```python
from build123d import *

# Parameters (mm, degrees)
F0_W     = 47.4027246237
F0_H     = 29.581496492
F1_DEPTH = 25
F3_D     = 5.5
F3_DEPTH = 12
F3_TIP   = 1.6523667023
F5_D     = 5.5
F5_DEPTH = 12
F5_TIP   = 1.6523667023


with BuildPart() as f1:
    # F0 (on Front) → F1 (new body)
    with BuildSketch(Plane.XZ):
        with Locations((23.7013623118, 14.790748246)):
            Rectangle(F0_W, F0_H)
    extrude(amount=F1_DEPTH)

    # F3
    with Locations(Plane.XY.offset(29.581496492)):
        with Locations((23.7013623118, -12.5)):
            Hole(F3_D / 2, depth=F3_DEPTH)
            with Locations((0, 0, -(F3_DEPTH + F3_TIP / 2))):  # 118° drill point
                Cone(0, F3_D / 2, F3_TIP, mode=Mode.SUBTRACT)

    # F5
    with Locations(Plane(origin=(0, 0, 0), x_dir=(-1, 0, 0), z_dir=(0, 1, 0))):
        with Locations((-39.530955255, 23.4460607171), (-30.8633740127, 23.4530330807), (-22.1957927704, 23.4600054443), (-13.5282115281, 23.4669778079), (-4.8606302857, 23.4739501715), (-39.530955255, 5.6460607171), (-39.530955255, 14.5460607171), (-4.8606302857, 5.6739501715), (-30.8633740127, 14.5530330807), (-4.8606302857, 14.5739501715), (-30.8633740127, 5.6530330807), (-22.1957927704, 14.5600054443), (-13.5282115281, 14.5669778079), (-22.1957927704, 5.6600054443), (-13.5282115281, 5.6669778079)):
            Hole(F5_D / 2, depth=F5_DEPTH)
            with Locations((0, 0, -(F5_DEPTH + F5_TIP / 2))):  # 118° drill point
                Cone(0, F5_D / 2, F5_TIP, mode=Mode.SUBTRACT)


solid = f1.part
```
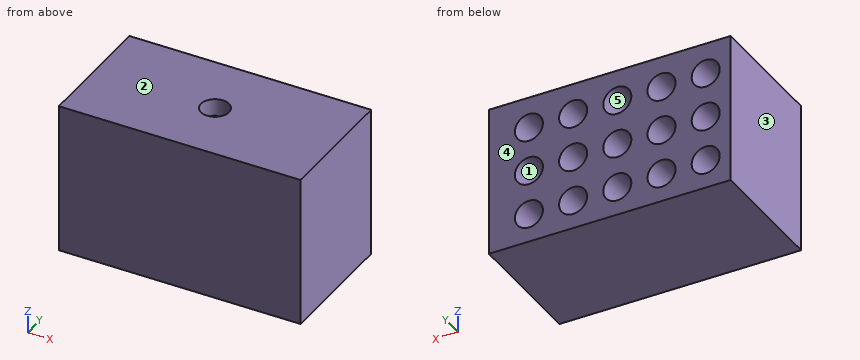
For this review, take the finished solid that the model builds, in its own axes (mm). Face numbers are marked on the shaded views. A direction names the side the tool comes from. Coordinates: 2 decimals unless noted, no trailing zeros. Answer as a JSON object with one key per item and string values. Group by question number.
1. We need section A-A on y = -3.5. Give the number of separate pieces and of enclosed holes in the cut face, then the cut area to 3 significant figures.
2. Clearance check with flat-ended pins moving along their axes: P1, Ø3.5, axis at x = 39.53, z = 14.55, coming from the +Y side; P2, Ø5, axis at x = 4.86, z = 5.67, coming from the +Y side; P3, Ø5, axis at x = 22.2, z = 23.46, coming from the +Y side. State where each tip first meets the part, or that it passes through.
3. The part is to be moulded in two halves that separate along Z. For the marked faces 1, 2 and 3, say which applies: pulls with the +Z half, pulls with the -Z half, needs draft (parallel to the pull), parting line crosses it, or undercut.
4. For the marked faces 4 and 5, list the 3-axis set-ups (+Z, -Z, +X, -X, +Y, -Y) from which the entire face can be reached by the end or side of a thin tool; tool diameter is ignored.
5. For probe 1 along Z at (x, y) = (11, -8.25); probe 2 along X at (y, z) = (-2, 16.5); probe 3 along Z at (x, y) = (39, -1.5), list the stretches that pass through material, from the lowest coordinate up.
Final values:
{
 "1": {"separate pieces": "1", "enclosed holes": "15", "area": "1,050 mm²"},
 "2": {"P1": "y = -12.6", "P2": "y = -12.15", "P3": "y = -12.15"},
 "3": {"face 1": "undercut", "face 2": "pulls with the +Z half", "face 3": "needs draft"},
 "4": {"face 4": "+Z, -Z, +X, -X, +Y", "face 5": "+Y"},
 "5": {"probe 1": "0 to 4.59, 6.75 to 13.49, 15.65 to 22.39, 24.55 to 29.58", "probe 2": "0 to 2.9, 6.82 to 11.57, 15.48 to 20.25, 24.14 to 28.92, 32.81 to 37.6, 41.47 to 47.4", "probe 3": "0 to 2.95, 8.34 to 11.85, 17.24 to 20.75, 26.14 to 29.58"}
}
